The figure shows three views and two pictorial views of one solid part (mm, origin at its lowest corner). Answer the questions. A direction names the side the tool comes from. Give positions to 0.01 mm unless a question says otherwise; leave off trailing zeros. Loops run counter-clockwise (first coordinate to the right, second up) from the corner with the lowest first, then second, coordinate; pieces in that order, holes last. Notation, with made-up numbers: M 22.5,38 L 27.5,38 A20 cw 27.5,61 Z; hole C 17,20 d11. An arc over 180 degrees is marked long. Answer in a Markdown table with one row per item. Add a question column.
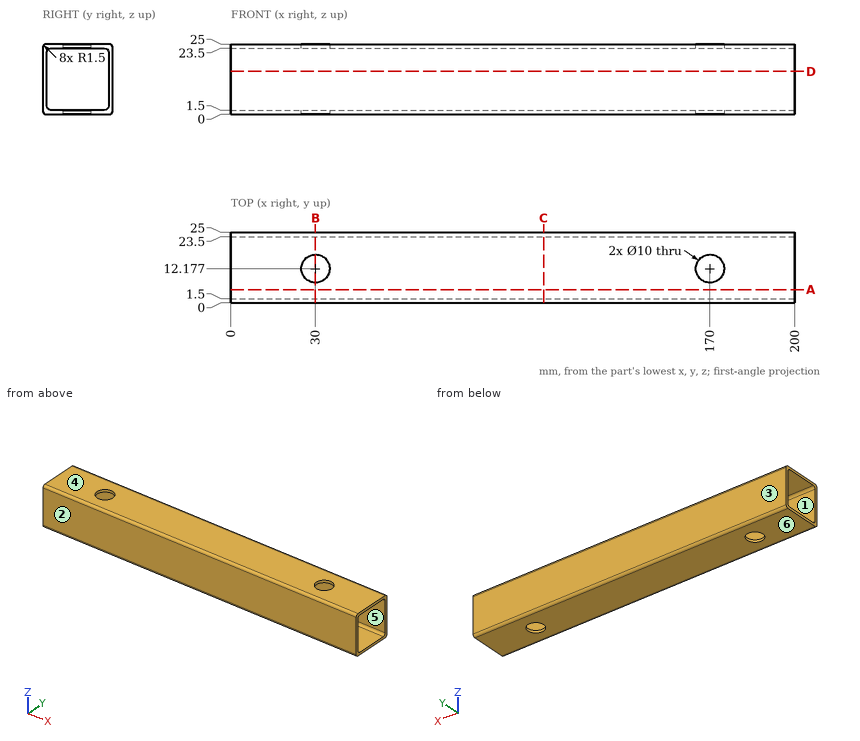
(1) Section C-C, the plane x = 111 is taken. Determine the outline of the cut face in (y, z), and give its area (3 significant figures).
(2) This flat-tipped pin is pushed along its axis until it touches: P1, Ø6, axis at x = 170, y = 12.18, coming from the -Z side. Where does it stop, or does it pass through?
(3) Section B-B, the plane x = 30 is taken. Determine the outline of the cut face in (y, z), and give its area (3 significant figures).
(4) Which of the six approach directions +Z, -Z, +X, -X, +Y, -Y give full straight-line access (tool end or side, diameter ignored) to the marked faces 1 and 2?
(5) Section A-A, the plane y = 4.75 is taken. Determine the outline of the cut face in (x, z).
(6) The mould has two halves that part along Z. Classify the marked faces 3, 4, 5 and 6: pulls with the +Z half, pulls with the -Z half, needs draft (parallel to the pull), parting line crosses it, or undercut.
(7) Consider line 1 along Z through (x, y) = (160, 12); line 2 along Y through (x, z) = (170, 24.3). Determine where each line is inside the solid, lowest interval first. Write a range as from..to.
Numbers:
| question | item | result |
|---|---|---|
| 1 | outline | M 0,1.5 A1.5 ccw 1.5,0 L 23.5,0 A1.5 ccw 25,1.5 L 25,23.5 A1.5 ccw 23.5,25 L 1.5,25 A1.5 ccw 0,23.5 Z; hole M 1.5,3 A1.5 ccw 3,1.5 L 22,1.5 A1.5 ccw 23.5,3 L 23.5,22 A1.5 ccw 22,23.5 L 3,23.5 A1.5 ccw 1.5,22 Z |
| 1 | area | 141 mm² |
| 2 | P1 | passes through |
| 3 | outline | M 0,1.5 A1.5 ccw 1.5,0 L 7.18,0 L 7.18,1.5 L 3,1.5 A1.5 cw 1.5,3 L 1.5,22 A1.5 cw 3,23.5 L 7.18,23.5 L 7.18,25 L 1.5,25 A1.5 ccw 0,23.5 Z; M 17.18,0 L 23.5,0 A1.5 ccw 25,1.5 L 25,23.5 A1.5 ccw 23.5,25 L 17.18,25 L 17.18,23.5 L 22,23.5 A1.5 cw 23.5,22 L 23.5,3 A1.5 cw 22,1.5 L 17.18,1.5 Z |
| 3 | area | 111 mm² |
| 4 | face 1 | +X, -X |
| 4 | face 2 | +Z, -Z, +X, -X, -Y |
| 5 | outline | M 0,0 L 200,0 L 200,1.5 L 0,1.5 Z; M 0,23.5 L 200,23.5 L 200,25 L 0,25 Z |
| 6 | face 3 | needs draft |
| 6 | face 4 | pulls with the +Z half |
| 6 | face 5 | undercut |
| 6 | face 6 | pulls with the -Z half |
| 7 | line 1 | z = 0..1.5, 23.5..25 |
| 7 | line 2 | y = 0.23..7.18, 17.18..24.77 |
